from build123d import *

# Parameters (mm, degrees)
F0_W          = 25.2043232322
F0_H          = 25.1512657851
F1_DEPTH      = 50
F1_DEPTH_BACK = 25
F2_W          = 24.7411523014
F2_H          = 25.458579883
F3_DEPTH      = 25
F3_DEPTH_BACK = 50
F4_W          = 25.3962129354
F4_H          = 25.0760298222
F5_DEPTH      = 25
F5_DEPTH_BACK = 50


with BuildPart() as f1:
    # F0 (on Front) → F1 (new body, two sides)
    with BuildSketch(Plane.XZ) as f1_sk:
        with Locations((12.6021616161, 12.5756328925)):
            Rectangle(F0_W, F0_H)
    extrude(amount=-F1_DEPTH)
    extrude(f1_sk.sketch, amount=F1_DEPTH_BACK)

    # F2 (on Top) → F3 (join, two sides)
    with BuildSketch(Plane.XY) as f3_sk:
        with Locations((12.3705761507, 12.7292899415)):
            Rectangle(F2_W, F2_H)
    extrude(amount=-F3_DEPTH)
    extrude(f3_sk.sketch, amount=F3_DEPTH_BACK)

    # F4 (on Right) → F5 (join, two sides)
    with BuildSketch(Plane.YZ) as f5_sk:
        with Locations((12.6981064677, 12.5380149111)):
            Rectangle(F4_W, F4_H)
    extrude(amount=-F5_DEPTH)
    extrude(f5_sk.sketch, amount=F5_DEPTH_BACK)


solid = f1.part
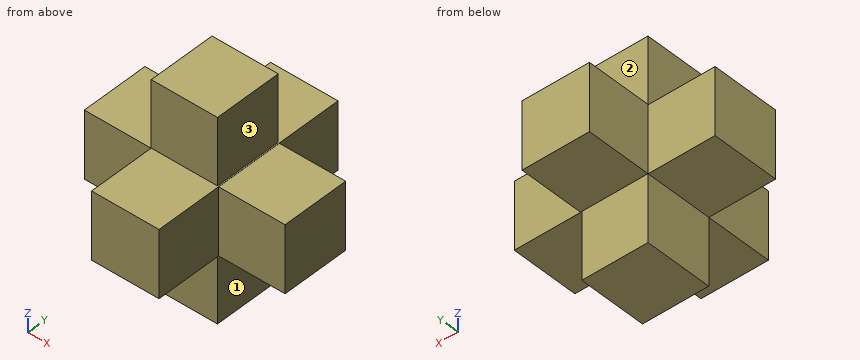
Part model, mm, in its own coordinate system. Face numbers are marked on the shaded views. A direction names the side the tool comes from. Give positions to 0.01 mm unless a question says otherwise; leave off trailing zeros. Order: outer loops, then holes, each group sorted by start corner. A loop starts at its lowest first (then second) coordinate and runs counter-clockwise, first axis right, second up. Notation, with made-up numbers: (78, -21.5) - (111, -21.5) arc R22 cw to (111, 0.5) - close; hole circle Ø8 at (40, 71.5). An arc over 180 degrees is marked (long way). One line per question, with ' | ' between items.
1. Band-saw the part on C-C on z = 9. List the corners of the cut face in (x, y), then the cut area to 3 significant figures.
Filled in:
outline: (-25, 0) - (0, 0) - (0, -25) - (25.2, -25) - (25.2, 0) - (50, 0) - (50, 25.4) - (25.2, 25.4) - (25.2, 50) - (0, 50) - (0, 25.4) - (-25, 25.4) - close | area: 3,150 mm²
2. Band-saw the part on D-D on x = 31. List the corners of the cut face in (y, z), then the cut area to 3 significant figures.
Filled in:
outline: (0, 0) - (25.4, 0) - (25.4, 25.08) - (0, 25.08) - close | area: 637 mm²
3. Band-saw the part on B-B on y = 21. List the corners of the cut face in (x, z).
Filled in:
outline: (-25, 0) - (0, 0) - (0, -25) - (24.74, -25) - (24.74, 0) - (50, 0) - (50, 25.08) - (25.2, 25.08) - (25.2, 25.15) - (24.74, 25.15) - (24.74, 50) - (0, 50) - (0, 25.08) - (-25, 25.08) - close
4. Drill centre lines: probe 1 along X at (y, z) = (1, -1.5); probe 2 along Y at (x, z) = (32, 20); probe 3 along Z at (x, y) = (42, 16.5). Where is each one in solid material? Low to high.
Filled in:
probe 1: 0 to 24.74 | probe 2: 0 to 25.4 | probe 3: 0 to 25.08
5. Band-saw the part on A-A on x = 1.5. List the corners of the cut face in (y, z), then the cut area to 3 significant figures.
Filled in:
outline: (-25, 0) - (0, 0) - (0, -25) - (25.46, -25) - (25.46, 0) - (50, 0) - (50, 25.15) - (25.46, 25.15) - (25.46, 50) - (0, 50) - (0, 25.15) - (-25, 25.15) - close | area: 3,160 mm²
6. Drop flat-ended pins along their axis: P1, Ø12, axis at x = 9, z = 38, coming from the +Y side; P2, Ø12.5, axis at x = -7.5, z = 16.5, coming from the +Y side; P3, Ø12, axis at y = 42, z = 0, coming from the -X side; P4, Ø20, axis at x = 6.5, z = -6.5, coming from the -Y side. Give the stop position or say it passes through.
Filled in:
P1: y = 25.46 | P2: y = 25.4 | P3: x = 0 | P4: y = -25
7. Which spindle directions (+Z, -Z, +X, -X, +Y, -Y) get a long thin tool onto all of the face, cutting with end or side? Do the marked faces 1, 2 and 3. Say none if no direction does.
Filled in:
face 1: -Z, +X, +Y, -Y | face 2: +Z, +X, -X, +Y | face 3: +Z, +X, +Y, -Y
